from build123d import *

# Parameters (mm, degrees)
SKETCH1_R           = 15
BOSS_EXTRUDE1_DEPTH = 6.4
CUT_EXTRUDE1_DEPTH  = 0.5
SKETCH3_R           = 2.5
BOSS_EXTRUDE2_DEPTH = 9
SKETCH4_R           = 3.8
CUT_EXTRUDE2_DEPTH  = 2
SKETCH6_R           = 4
BOSS_EXTRUDE3_DEPTH = 1
SKETCH5_R           = 2.5
CUT_EXTRUDE3_DEPTH  = 6.4
SKETCH8_W           = 12
SKETCH8_H           = 3.25
BOSS_EXTRUDE4_DEPTH = 4
SKETCH9_R           = 2.5
BOSS_EXTRUDE6_DEPTH = 11


with BuildPart() as part:
    # Sketch1 → Boss-Extrude1 (new body)
    with BuildSketch(Plane(origin=(0, 0, 0), x_dir=(1, 0, 0), z_dir=(0, 1, 0))):
        Circle(SKETCH1_R)
    extrude(amount=BOSS_EXTRUDE1_DEPTH)

    # Sketch2 → Cut-Extrude1 (cut)
    with BuildSketch(Plane(origin=(0, 6.4, 0), x_dir=(1, 0, 0), z_dir=(0, 1, 0))):
        with BuildLine():
            ThreePointArc((-5.083306011, -1.5), (0, -5.3), (5.083306011, -1.5))
            Line((5.083306011, -1.5), (11.805083651, -1.5))
            ThreePointArc((11.805083651, -1.5), (0, -11.9), (-11.805083651, -1.5))
            Line((-11.805083651, -1.5), (-5.083306011, -1.5))
        make_face()
        with BuildLine():
            Line((-11.805083651, 1.5), (-5.083306011, 1.5))
            ThreePointArc((-5.083306011, 1.5), (0, 5.3), (5.083306011, 1.5))
            Line((5.083306011, 1.5), (11.805083651, 1.5))
            ThreePointArc((11.805083651, 1.5), (0, 11.9), (-11.805083651, 1.5))
        make_face()
    extrude(amount=-CUT_EXTRUDE1_DEPTH, mode=Mode.SUBTRACT)

    # Sketch3 → Boss-Extrude2 (add)
    with BuildSketch(Plane(origin=(0, 5.9, 0), x_dir=(1, 0, 0), z_dir=(0, 1, 0))):
        with Locations((0, -10)):
            Circle(SKETCH3_R)
        with Locations((0, 10)):
            Circle(SKETCH3_R)
    extrude(amount=BOSS_EXTRUDE2_DEPTH)

    # Sketch4 → Cut-Extrude2 (cut)
    with BuildSketch(Plane(origin=(0, 6.4, 0), x_dir=(1, 0, 0), z_dir=(0, 1, 0))):
        Circle(SKETCH4_R)
    extrude(amount=-CUT_EXTRUDE2_DEPTH, mode=Mode.SUBTRACT)

    # Sketch6 → Boss-Extrude3 (add)
    with BuildSketch(Plane.XZ):
        Circle(SKETCH6_R)
    extrude(amount=BOSS_EXTRUDE3_DEPTH)

    # Sketch5 → Cut-Extrude3 (cut, through all)
    with BuildSketch(Plane(origin=(0, 4.4, 0), x_dir=(1, 0, 0), z_dir=(0, 1, 0))):
        Circle(SKETCH5_R)
    extrude(amount=-CUT_EXTRUDE3_DEPTH, mode=Mode.SUBTRACT)

    # Sketch8 → Boss-Extrude4 (add)
    with BuildSketch(Plane(origin=(0, 2, 0), x_dir=(1, 0, 0), z_dir=(0, 1, 0))):
        with Locations((-19, 4.125)):
            Rectangle(SKETCH8_W, SKETCH8_H)
        with Locations((-19, -4.125)):
            Rectangle(SKETCH8_W, SKETCH8_H)
    extrude(amount=BOSS_EXTRUDE4_DEPTH)

    # Sketch9 → Boss-Extrude6 (add, symmetric)
    with BuildSketch(Plane.XY):
        with Locations((-25, 3.5)):
            Circle(SKETCH9_R)
    extrude(amount=BOSS_EXTRUDE6_DEPTH, both=True)


solid = part.part
Read the model definition and answer for the solid it produces. Units are mm, in the model's axes. A direction names the side the tool comes from. Give positions to 0.01 mm unless a question says otherwise; leave off trailing zeros. Write each loop counter-clockwise with the first axis right and the second up, starting at its lowest first coordinate (ties: lowest second). Pieces come first, ordered by that corner, then holes. Notation, with made-up numbers: (-12, 0) -> (11, 0) arc R4 ccw to (11, 4) -> close; hole circle Ø8 at (86, 67.25). An arc over 180 degrees is marked (long way). Answer as a JSON object with one key per item and string values. Group by question number.
1) Each of these flat-tipped pins is pushed along its axis until it touches: P1, Ø0.6, axis at x = 10, y = 6, coming from the -Z side; P2, Ø8.5, axis at x = -1.5, z = 1, coming from the +Y side; P3, Ø6, axis at x = -23, z = -10, coming from the +Y side. Where does it stop, or does it pass through?
2) The mould has two halves that part along Z. Classify faces 5 (the cylindrical face through (-3.796, 5.414, -0.167)), 6 (the cylindrical face through (-0.867, -0.493, -3.905)), 7 (the flat face through (-18, 4, 5.75)), 8 (the flat face through (0, 14.9, -10)): +Z half, -Z half, draft (parallel to the pull), parting line (faces both ways), or undercut.
3) Find section B-B (y = 1.5). Write down the section's boundary in (x, z).
4) A tool of negligible diameter and unlimited length cuts with its end or side. For faces 1 (the flat face through (0, 5.9, 7)), 2 (the flat face through (-25, 4, -11)), 3 (the flat face through (3, 0, 3)), 4 (the cylindrical face through (-27.5, 3.6, 0.2)), from which of +Z, -Z, +X, -X, +Y, -Y can it reach the whole face along a straight path? Write none if from no direction.
5) Find section C-C (x = 0). Write down the section's boundary in (y, z), and give its area (3 significant figures).
6) Consider L1, parallel to Z at x = 0, y = 6; L2, parallel to Z at x = -21, y = 3; L3, parallel to Z at x = 0, y = 5.55. Determine where each line is inside the solid, lowest interval first. Write a range as from..to.
7) Find section A-A (z = 0). Write down the section's boundary in (x, y), and give its area (3 significant figures).
8) Find section D-D (z = 10). Write down the section's boundary in (x, y).
Values follow:
{
 "1": {"P1": "stops at z = -11.44", "P2": "stops at y = 6.4", "P3": "stops at y = 6"},
 "2": {"face 5": "undercut", "face 6": "parting line", "face 7": "+Z half", "face 8": "draft"},
 "3": {"outline": "(-26.5, -11) -> (-23.5, -11) -> (-23.5, 11) -> (-26.5, 11) -> close; circle Ø30 at (0, 0); hole circle Ø5 at (0, 0)"},
 "4": {"face 1": "+Y", "face 2": "-Z, -X, +Y, -Y", "face 3": "-Y", "face 4": "none"},
 "5": {"outline": "(-1, -4) -> (0, -4) -> (0, -15) -> (6.4, -15) -> (6.4, -12.5) -> (14.9, -12.5) -> (14.9, -7.5) -> (5.9, -7.5) -> (5.9, -5.3) -> (6.4, -5.3) -> (6.4, -3.8) -> (4.4, -3.8) -> (4.4, -2.5) -> (-1, -2.5) -> close; (-1, 2.5) -> (4.4, 2.5) -> (4.4, 3.8) -> (6.4, 3.8) -> (6.4, 5.3) -> (5.9, 5.3) -> (5.9, 7.5) -> (14.9, 7.5) -> (14.9, 12.5) -> (6.4, 12.5) -> (6.4, 15) -> (0, 15) -> (0, 4) -> (-1, 4) -> close", "area": "241 mm2"},
 "6": {"L1": "z = -15..-7.5, -5.3..-3.8, 3.8..5.3, 7.5..15", "L2": "z = -5.75..-2.5, 2.5..5.75", "L3": "z = -15..-3.8, 3.8..15"},
 "7": {"outline": "circle Ø5 at (-25, 3.5); (-15, 0) -> (-4, 0) -> (-4, -1) -> (-2.5, -1) -> (-2.5, 4.4) -> (-3.8, 4.4) -> (-3.8, 6.4) -> (-15, 6.4) -> close; (2.5, -1) -> (4, -1) -> (4, 0) -> (15, 0) -> (15, 6.4) -> (3.8, 6.4) -> (3.8, 4.4) -> (2.5, 4.4) -> close", "area": "177 mm2"},
 "8": {"outline": "circle Ø5 at (-25, 3.5); (-11.18, 0) -> (11.18, 0) -> (11.18, 6.4) -> (6.45, 6.4) -> (6.45, 5.9) -> (2.5, 5.9) -> (2.5, 14.9) -> (-2.5, 14.9) -> (-2.5, 5.9) -> (-6.45, 5.9) -> (-6.45, 6.4) -> (-11.18, 6.4) -> close"}
}
